The model under review builds one solid part; all positions refer to its coordinate system, in mm. Face numbers are marked on the shaded views. A direction names the side the tool comes from. Coordinates: 2 decimals unless noted, no trailing zeros. Loops run counter-clockwise (first coordinate to the right, second up) from the corner with the lowest first, then second, coordinate; pieces in that order, holes last. Notation, with made-up numbers: M 48.5,-37 L 55.5,-37 A27 cw 55.5,-5 Z; hole C 83.5,-4.75 d2. An arc over 180 degrees is marked long. Use CSV: the item, a comma, the result in double quotes. Start each with the question number.
1. Draft analysis for pull direction X (two halves, no side actions). For the marked faces 1, 2 and 3, state which applies: +X half, -X half, draft (parallel to the pull), parting line (faces both ways), or undercut.
2. Add section A-A, the plane z = -19.5. Write out the cut boundary in (x, y).
3. Add section C-C, the plane y = 9. Write out the cut boundary in (x, z).
4. Tool access review of the marked faces 4 and 5: name each direction out of +Z, -Z, +X, -X, +Y, -Y from which nothing blocks a thin tool from reaching the whole face with its end or side.
5. For L1, parallel to Z at x = 84, y = 39.5; L2, parallel to X at y = 48.5, z = -40.5; L3, parallel to Y at x = -13, z = 6.5, list the stretches that pass through material, from the lowest coordinate up.
6. Add section B-B, the plane x = 37. Write out the cut boundary in (y, z).
from build123d import *

# Parameters (mm, degrees)
SKETCH1_W           = 200
SKETCH1_H           = 120
BOSS_EXTRUDE1_DEPTH = 50
SHELL2_T            = -2
FILLET1_R           = 2


with BuildPart() as part:
    # Sketch1 → Boss-Extrude1 (new body)
    with BuildSketch(Plane(origin=(0, 0, 0), x_dir=(1, 0, 0), z_dir=(0, 1, 0))):
        Rectangle(SKETCH1_W, SKETCH1_H)
    extrude(amount=BOSS_EXTRUDE1_DEPTH)

    # Shell2
    shell2_openings = [part.faces().sort_by_distance(p)[0] for p in [
        (0, 50, 0),
    ]]
    offset(amount=SHELL2_T, openings=shell2_openings, kind=Kind.INTERSECTION)

    # Fillet1
    fillet1_edges = [part.edges().sort_by_distance(p)[0] for p in [
        (0, 0, 60),
        (-100, 0, 0),
        (0, 0, -60),
        (100, 0, 0),
        (100, 25, 60),
        (-100, 25, 60),
        (-100, 25, -60),
        (100, 25, -60),
    ]]
    fillet(fillet1_edges, radius=FILLET1_R)


solid = part.part
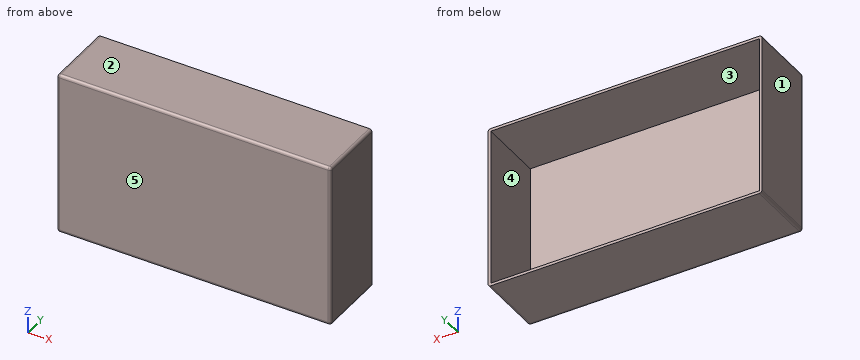
Computed:
1,face 1,"-X half"
1,face 2,"draft"
1,face 3,"undercut"
2,outline,"M -100,2 A2 ccw -98,0 L 98,0 A2 ccw 100,2 L 100,50 L 98,50 L 98,2 L -98,2 L -98,50 L -100,50 Z"
3,outline,"M -100,-58 A2 ccw -98,-60 L 98,-60 A2 ccw 100,-58 L 100,58 A2 ccw 98,60 L -98,60 A2 ccw -100,58 Z; hole M -98,-58 L 98,-58 L 98,58 L -98,58 Z"
4,face 4,"+Y"
4,face 5,"+Z, -Z, +X, -X, -Y"
5,L1,"z = -60 to -58, 58 to 60"
5,L2,"x = -100 to -98, 98 to 100"
5,L3,"y = 0 to 2"
6,outline,"M 0,-58 A2 ccw 2,-60 L 50,-60 L 50,-58 L 2,-58 L 2,58 L 50,58 L 50,60 L 2,60 A2 ccw 0,58 Z"
